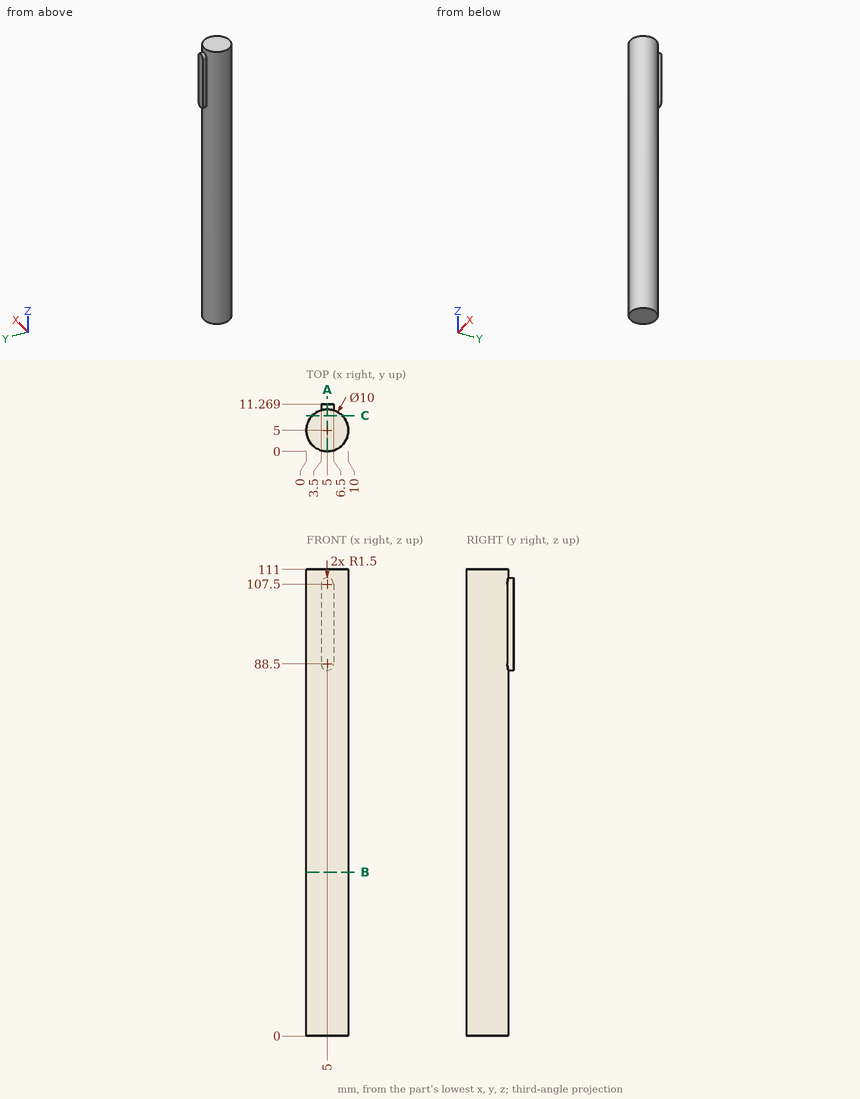
Here's the drawing with two shaded views (mm, measured from the low corner). I have some questions. Round coordinates to 2 decimals unless told otherwise and drop trailing zeros. Order: outer loops, then holes, each group sorted by start corner. A loop starts at its lowest first (then second) coordinate and runs counter-clockwise, first axis right, second up. Notation, with made-up numbers: (66.5, 84.5) -> (118.5, 84.5) arc R33 cw to (118.5, 118.5) -> close; hole circle Ø2 at (-25, 26.5). An arc over 180 degrees is marked (long way). Write each question's results on one line, items separated by ' | '. Start each with the question number.
Item 1: Will these pins go through, and if not, where does the flat tip stop? pin 1 (2 mm diameter, centred on y = 7.5, z = 66, fed in from -X); pin 2 (1 mm diameter, centred on x = 6, z = 31.5, fed in from +Y); pin 3 (1.5 mm diameter, centred on y = 9, z = 95.5, fed in from +X).
Item 2: If we section it at B-B, the plane z = 39: Write out the boundary of the cut face in (x, y), then the cut area to 3 significant figures.
Item 3: Please list where these lines run through material, in increasing order: L1, parallel to Y at x = 4.75, z = 41.5; L2, parallel to X at y = 6.75, z = 75; L3, parallel to Z at x = 4.5, y = 10.25.
Item 4: If we section it at A-A, the plane x = 5: Write out the boundary of the cut face in (y, z), then the cut area to 3 significant figures.
Item 5: If we section it at C-C, the plane y = 8.5: Write out the boundary of the cut face in (x, z), then the cut area to 3 significant figures.
Results:
1) pin 1: stops at x = 0.23 | pin 2: stops at y = 9.97 | pin 3: stops at x = 8.8
2) outline: circle Ø10 at (5, 5) | area: 78.5 mm2
3) L1: y = 0.01 to 9.99 | L2: x = 0.32 to 9.68 | L3: z = 87.09 to 108.91
4) outline: (0, 0) -> (10, 0) -> (10, 87) -> (11.27, 87) -> (11.27, 109) -> (10, 109) -> (10, 111) -> (0, 111) -> close | area: 1,140 mm2
5) outline: (1.43, 0) -> (8.57, 0) -> (8.57, 111) -> (1.43, 111) -> close | area: 793 mm2
